from build123d import *

# Parameters (mm, degrees)
BOSS_EXTRUDE1_DEPTH     = 20.32
SHELL1_T                = -2.54
SKETCH3_R               = 6.35
BOSS_EXTRUDE2_DEPTH     = 2.54
SKETCH5_R               = 0.635
CUT_EXTRUDE2_DEPTH      = 1
CUT_EXTRUDE2_DEPTH_BACK = 21.32


with BuildPart() as part:
    # Sketch2 → Boss-Extrude1 (new body)
    with BuildSketch(Plane(origin=(0, 0, 0), x_dir=(0, 0, -1), z_dir=(1, 0, 0))):
        with BuildLine():
            Line((0, 0), (38.1, 0))
            Line((38.1, 0), (38.1, -6.35))
            ThreePointArc((38.1, -6.35), (34.505388745, -9.09166098), (33.149673366, -13.404429327))
            Line((33.149673366, -13.404429327), (33.149673366, -20.32))
            Line((33.149673366, -20.32), (25.753107907, -20.32))
            ThreePointArc((25.753107907, -20.32), (12.259334003, -17.809647323), (0, -11.637732342))
            Line((0, -11.637732342), (0, 0))
        make_face()
    extrude(amount=BOSS_EXTRUDE1_DEPTH)

    # Shell1
    shell1_openings = [part.faces().sort_by_distance(p)[0] for p in [
        (10.16, -3.175, -38.1),
        (10.16, -9.484437822, -35.065112714),
        (10.16, -16.862214664, -33.149673366),
        (10.16, -20.32, -29.451390636),
        (10.16, -16.894256747, -12.567943978),
        (10.16, -5.818866171, 0),
    ]]
    offset(amount=SHELL1_T, openings=shell1_openings, kind=Kind.INTERSECTION)

    # Sketch3 → Boss-Extrude2 (add)
    with BuildSketch(Plane(origin=(0, 0, 0), x_dir=(1, 0, 0), z_dir=(0, 1, 0))):
        with Locations((10.16, 7.62)):
            Circle(SKETCH3_R)
    extrude(amount=BOSS_EXTRUDE2_DEPTH)

    # Sketch5 → Cut-Extrude2 (cut, two sides)
    with BuildSketch(Plane(origin=(20.32, 0, 0), x_dir=(0, 0, -1), z_dir=(1, 0, 0))) as cut_extrude2_sk:
        with Locations((25.529673366, -15.24)):
            Circle(SKETCH5_R)
    extrude(amount=CUT_EXTRUDE2_DEPTH, mode=Mode.SUBTRACT)
    extrude(cut_extrude2_sk.sketch, amount=-CUT_EXTRUDE2_DEPTH_BACK, mode=Mode.SUBTRACT)


solid = part.part
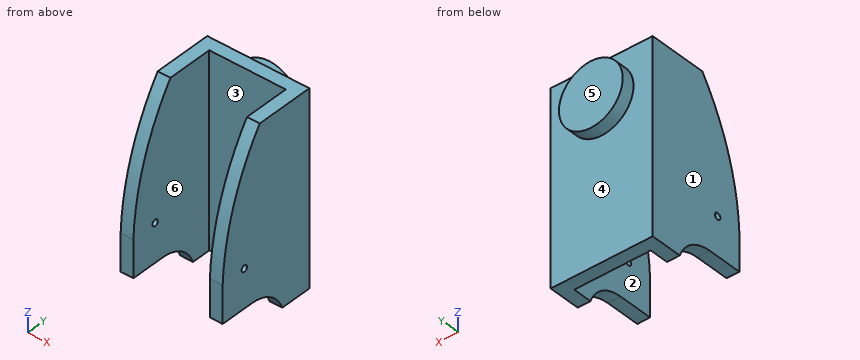
For this review, take the finished solid that the model builds, in its own axes (mm). Face numbers are marked on the shaded views. A direction names the side the tool comes from. Round coordinates to 2 decimals unless told otherwise and drop trailing zeros. Order: outer loops, then holes, each group sorted by start corner. A loop starts at its lowest first (then second) coordinate and runs counter-clockwise, first axis right, second up. Notation, with made-up numbers: (31, -8.75) -> (64, -8.75) arc R17 ccw to (64, 16.25) -> close; hole circle Ø2 at (11, 56.25). An arc over 180 degrees is marked (long way). Write item = value, one per line. Start each with the question number.
1) Take a section at A-A on y = -5. State the section outline as (x, z) points.
2) To check wall thickness, follow line 1 (X direction, y = -7, z = -9); line 2 (Y direction, x = 14.5, z = -23.5); line 3 (Y direction, x = 2.5, z = -1.5). State the ranges of each line that lie inside material, in increasing order. Write a range as from..to.
3) Tool access review of the marked faces 5 and 6: name each direction out of +Z, -Z, +X, -X, +Y, -Y from which nothing blocks a thin tool from reaching the whole face with its end or side.
4) Take a section at C-C on y = -15.24. State the section outline as (x, z) points, plus the area to 3 significant figures.
5) Take a section at D-D on x = 10.16. State the section outline as (y, z) points.
6) Take a section at B-B on z = -29. State the section outline as (x, y) points, plus the area to 3 significant figures.
7) The part is to be moulded in two halves that separate along X. For the marked faces 1, 2, 3 and 4, say which applies: +X half, -X half, draft (parallel to the pull), parting line (faces both ways), or undercut.
8) Insertion check: pin 1 (6 mm diameter, centred on x = 13.5, y = -3.5, fed in from +Z); pin 2 (7.5 mm diameter, centred on x = 8, z = -10.5, fed in from -Y); pin 3 (6 mm diameter, centred on x = 4.5, z = -20.5, fed in from +Y); pin 4 (0.8 mm diameter, centred on x = 2, y = -18, fed in from -Z). Each pin has a flat end and moves straight along its axis. Give the tip position at first contact, or say it passes through.
Verdict:
q1.outline = (0, -38.1) -> (2.54, -38.1) -> (2.54, 0) -> (0, 0) -> close; (17.78, -38.1) -> (20.32, -38.1) -> (20.32, 0) -> (17.78, 0) -> close
q2.line_1 = 0..2.54, 17.78..20.32
q2.line_2 = -2.54..0
q2.line_3 = -12.64..0
q3.face_5 = +Z, -Z, +X, -X, +Y
q3.face_6 = +Z, -Z, -Y
q4.outline = (0, -33.15) -> (2.54, -33.15) -> (2.54, -26.16) -> (0, -26.16) -> close; (0, -24.89) -> (2.54, -24.89) -> (2.54, -6.08) -> (0, -6.08) -> close; (17.78, -33.15) -> (20.32, -33.15) -> (20.32, -26.16) -> (17.78, -26.16) -> close; (17.78, -24.89) -> (20.32, -24.89) -> (20.32, -6.08) -> (17.78, -6.08) -> close
q4.area = 131 mm2
q5.outline = (-2.54, -38.1) -> (0, -38.1) -> (0, -13.97) -> (2.54, -13.97) -> (2.54, -1.27) -> (0, -1.27) -> (0, 0) -> (-2.54, 0) -> close
q6.outline = (0, -20.32) -> (2.54, -20.32) -> (2.54, -2.54) -> (17.78, -2.54) -> (17.78, -20.32) -> (20.32, -20.32) -> (20.32, 0) -> (0, 0) -> close
q6.area = 142 mm2
q7.face_1 = -X half
q7.face_2 = undercut
q7.face_3 = undercut
q7.face_4 = draft
q8.pin_1 = 0
q8.pin_2 = -2.54
q8.pin_3 = 0
q8.pin_4 = -33.15
